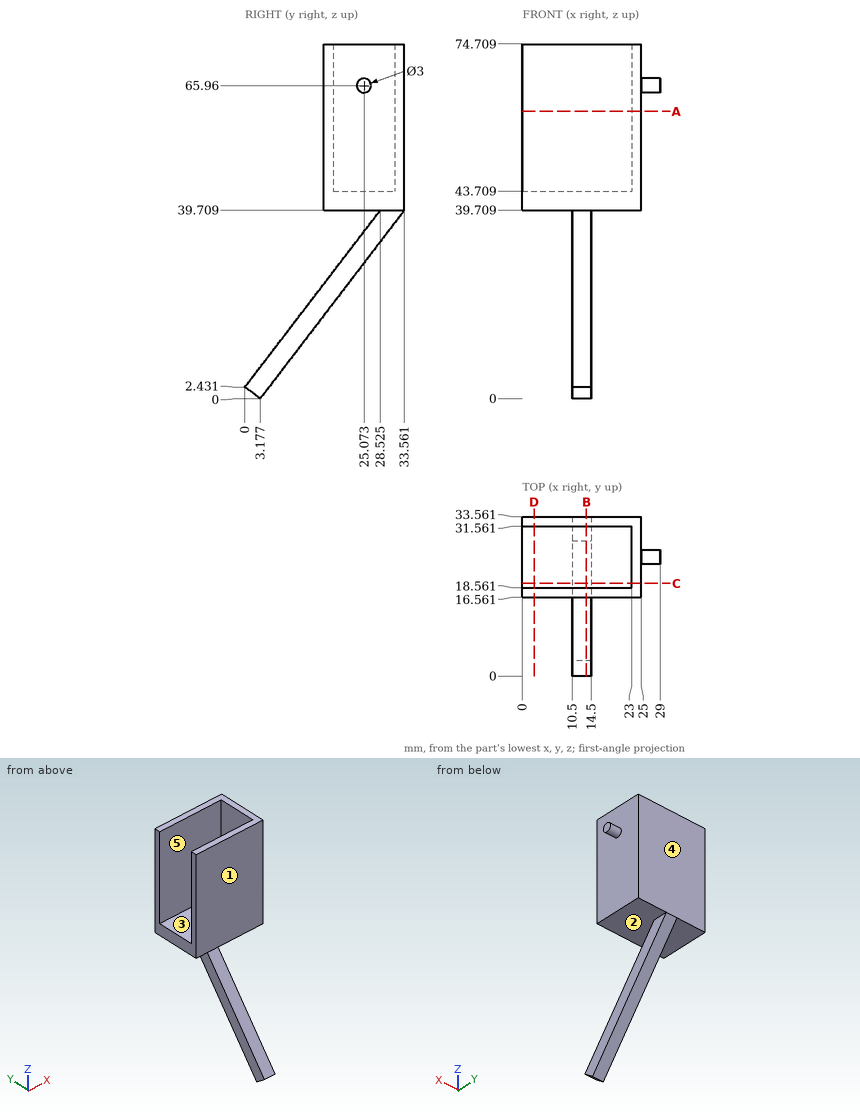
For this review, use the dimensioned drawing (mm, ordinates from the lowest corner) and the shaded views. A direction names the side the tool comes from. Coordinates: 2 decimals unless noted, no trailing zeros. Order: outer loops, then holes, each group sorted by start corner. A loop starts at its lowest first (then second) coordinate and runs counter-clockwise, first axis right, second up. Notation, with made-up numbers: M 51,87.5 L 59,87.5 A6 ccw 59,94.5 Z; hole C 6.5,87 d6. An arc over 180 degrees is marked long. Answer as a JSON object with one key per item and string values. Group by question number.
1) Add section D-D, the plane x = 2.5. Write out the cut boundary in (y, z), then the cut area to 3 significant figures.
2) For pin 1 (8.5 mm diameter, centred on x = 8, y = 24.5, fed in from -Z) (1 decimal); pin 2 (6.5 mm diameter, centred on x = 7, y = 25, fed in from +Z); pin 3 (1 mm diameter, centred on y = 16, z = 50, fed in from +X); pin 4 (11.5 mm diameter, centred on x = 14.5, z = 51.5, fed in from -Y), all flat-tipped, find the tip position at first contact; note any pin that passes through.
3) Tool access review of the marked faces 4 and 5: name each direction out of +Z, -Z, +X, -X, +Y, -Y from which nothing blocks a thin tool from reaching the whole face with its end or side.
4) Wall thickness on L1, parallel to Y at x = 2.25, z = 41.5; L2, parallel to Z at x = 5.5, y = 18.5; L3, parallel to X at y = 20, z = 46.5: over which ranges is each line inside the solid? List them lowest first.
5) Add section A-A, the plane z = 60.5. Write out the cut boundary in (x, y), then the cut area to 3 significant figures.
6) Add section B-B, the plane x = 13.5. Write out the cut boundary in (y, z) (1 decimal), then the cut area to 3 significant figures.
7) Mouldability with a two-part tool opening along Y and no side actions: class the marked faces 1, 2 and 3 as pulls with the +Y half, pulls with the -Y half, needs draft (parallel to the pull), parting line crosses it, or undercut.
8) Add section C-C, the plane y = 19.5. Write out the cut boundary in (x, z) (1 decimal).
Computed values:
{
 "1": {"outline": "M 16.56,39.71 L 33.56,39.71 L 33.56,74.71 L 31.56,74.71 L 31.56,43.71 L 18.56,43.71 L 18.56,74.71 L 16.56,74.71 Z", "area": "192 mm^2"},
 "2": {"pin 1": "stops at z = 23.4", "pin 2": "stops at z = 43.71", "pin 3": "passes through", "pin 4": "stops at y = 16.56"},
 "3": {"face 4": "+Z, -Z, +X, -X, +Y", "face 5": "+Z, -X"},
 "4": {"L1": "y = 16.56 to 33.56", "L2": "z = 39.71 to 74.71", "L3": "x = 23 to 25"},
 "5": {"outline": "M 0,16.56 L 25,16.56 L 25,33.56 L 0,33.56 L 0,31.56 L 23,31.56 L 23,18.56 L 0,18.56 Z", "area": "126 mm^2"},
 "6": {"outline": "M 0,2.4 L 3.2,0 L 33.6,39.7 L 33.6,74.7 L 31.6,74.7 L 31.6,43.7 L 18.6,43.7 L 18.6,74.7 L 16.6,74.7 L 16.6,39.7 L 28.5,39.7 Z", "area": "386 mm^2"},
 "7": {"face 1": "pulls with the -Y half", "face 2": "needs draft", "face 3": "undercut"},
 "8": {"outline": "M 0,39.7 L 25,39.7 L 25,74.7 L 23,74.7 L 23,43.7 L 0,43.7 Z; M 10.5,21.3 L 14.5,21.3 L 14.5,27.9 L 10.5,27.9 Z"}
}
